Could you check a few things on this model? Use its own coordinates, in mm. Face numbers are marked on the shaded views. A direction names the side the tool comes from. Give positions to 0.01 mm unless a question says otherwise; leave off trailing zeros. Write each loop counter-clockwise with the first axis right and the second up, starting at its lowest first coordinate (ties: lowest second). Pieces come first, ordered by that corner, then holes. Notation, with made-up numbers: M 11.5,62.25 L 42.5,62.25 A24 ccw 42.5,86.25 Z; hole C 26.25,28 d2. An arc over 180 degrees is marked long. Answer as a JSON object with one key per item and string values. Group by question number.
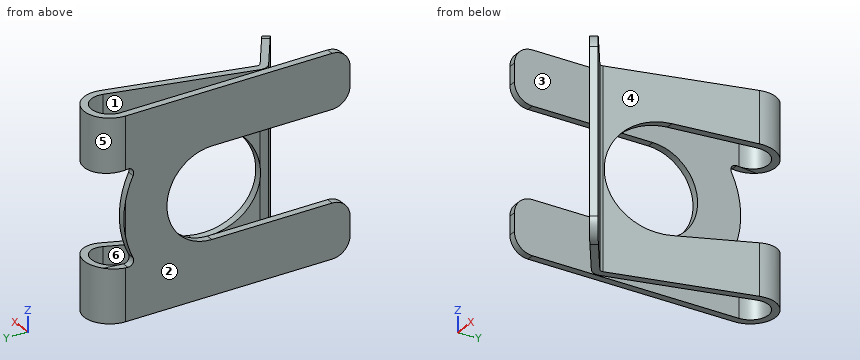
```python
from build123d import *

# Parameters (mm, degrees)
BOSS_EXTRUDE1_DEPTH      = 5.5
BOSS_EXTRUDE1_DEPTH_BACK = 5.5
CUT_EXTRUDE1_DEPTH       = 0.4
CUT_EXTRUDE2_DEPTH       = 3.8
CUT_EXTRUDE3_DEPTH       = 3.8
CUT_EXTRUDE4_DEPTH       = 0.4
CUT_EXTRUDE5_DEPTH       = 0.4
CUT_EXTRUDE6_DEPTH       = 0.4
CUT_EXTRUDE7_DEPTH       = 0.4
CUT_EXTRUDE8_DEPTH       = 0.8
CUT_EXTRUDE8_DEPTH_BACK  = 0.8


with BuildPart() as part:
    # Sketch1 → Boss-Extrude1 (new body, two sides)
    with BuildSketch(Plane.XY) as boss_extrude1_sk:
        with BuildLine():
            Line((0, 4.8), (0, -7.7))
            Line((0, -7.7), (0.4, -7.7))
            Line((0.4, -7.7), (0.4, 4.8))
            ThreePointArc((0.4, 4.8), (1.523848484, 5.79230114), (2.369323106, 4.554210017))
            Line((2.369323106, 4.554210017), (0.462124676, -2.967217351))
            ThreePointArc((0.462124676, -2.967217351), (0.483070792, -3.328406344), (0.707868785, -3.611888427))
            Line((0.707868785, -3.611888427), (3.611166589, -5.573025933))
            Line((3.611166589, -5.573025933), (3.835066425, -5.241561209))
            Line((3.835066425, -5.241561209), (0.931768621, -3.280423703))
            ThreePointArc((0.931768621, -3.280423703), (0.856835957, -3.185929675), (0.849853918, -3.065533344))
            Line((0.849853918, -3.065533344), (2.757052349, 4.455894023))
            ThreePointArc((2.757052349, 4.455894023), (1.573387877, 6.189221596), (0, 4.8))
        make_face()
    extrude(amount=BOSS_EXTRUDE1_DEPTH)
    extrude(boss_extrude1_sk.sketch, amount=-BOSS_EXTRUDE1_DEPTH_BACK)

    # Sketch2 → Cut-Extrude1 (cut)
    with BuildSketch(Plane(origin=(0, 0, 0), x_dir=(0, 0, -1), z_dir=(1, 0, 0))):
        with BuildLine():
            Line((-2.5, 0), (-2.5, -7.7))
            Line((-2.5, -7.7), (2.5, -7.7))
            Line((2.5, -7.7), (2.5, 0))
            ThreePointArc((2.5, 0), (0, 2.5), (-2.5, 0))
        make_face()
    extrude(amount=CUT_EXTRUDE1_DEPTH, mode=Mode.SUBTRACT)

    # Sketch3 → Cut-Extrude2 (cut)
    with BuildSketch(Plane(origin=(0.4, 0, 0), x_dir=(0, 0, -1), z_dir=(1, 0, 0))):
        with BuildLine():
            Line((2.989896199, 0.246009597), (2.5, 6.2))
            Line((2.5, 6.2), (-2.5, 6.2))
            Line((-2.5, 6.2), (-2.989896199, 0.246009597))
            ThreePointArc((-2.989896199, 0.246009597), (0, -3), (2.989896199, 0.246009597))
        make_face()
    extrude(amount=CUT_EXTRUDE2_DEPTH, mode=Mode.SUBTRACT)

    # Sketch4 → Cut-Extrude3 (cut)
    with BuildSketch(Plane(origin=(0.4, 0, 0), x_dir=(0, 0, -1), z_dir=(1, 0, 0))):
        with BuildLine():
            Line((2.62546601, 4.675139381), (2.5, 6.2))
            Line((2.5, 6.2), (-2.5, 6.2))
            Line((-2.5, 6.2), (-2.62546601, 4.675139381))
            ThreePointArc((-2.62546601, 4.675139381), (-2.494509309, 4.402012893), (-2.192256609, 4.382238122))
            ThreePointArc((-2.192256609, 4.382238122), (-6e-09, 4.9), (2.192256599, 4.382238127))
            ThreePointArc((2.192256599, 4.382238127), (2.494509304, 4.402012889), (2.62546601, 4.675139381))
        make_face()
    extrude(amount=-CUT_EXTRUDE3_DEPTH, mode=Mode.SUBTRACT)

    # Sketch5 → Cut-Extrude4 (cut)
    with BuildSketch(Plane(origin=(0, 0, 0), x_dir=(0, 0, -1), z_dir=(1, 0, 0))):
        with BuildLine():
            Line((-5.5, -7.7), (-4.5, -7.7))
            ThreePointArc((-4.5, -7.7), (-5.207106781, -7.407106781), (-5.5, -6.7))
            Line((-5.5, -6.7), (-5.5, -7.7))
        make_face()
    extrude(amount=CUT_EXTRUDE4_DEPTH, mode=Mode.SUBTRACT)

    # Sketch6 → Cut-Extrude5 (cut)
    with BuildSketch(Plane(origin=(0, 0, 0), x_dir=(0, 0, -1), z_dir=(1, 0, 0))):
        with BuildLine():
            Line((4.5, -7.7), (5.5, -7.7))
            Line((5.5, -7.7), (5.5, -6.7))
            ThreePointArc((5.5, -6.7), (5.207106781, -7.407106781), (4.5, -7.7))
        make_face()
    extrude(amount=CUT_EXTRUDE5_DEPTH, mode=Mode.SUBTRACT)

    # Sketch7 → Cut-Extrude6 (cut)
    with BuildSketch(Plane(origin=(0, 0, 0), x_dir=(0, 0, -1), z_dir=(1, 0, 0))):
        with BuildLine():
            Line((2.5, -7.7), (3.5, -7.7))
            ThreePointArc((3.5, -7.7), (2.792893219, -7.407106781), (2.5, -6.7))
            Line((2.5, -6.7), (2.5, -7.7))
        make_face()
    extrude(amount=CUT_EXTRUDE6_DEPTH, mode=Mode.SUBTRACT)

    # Sketch8 → Cut-Extrude7 (cut)
    with BuildSketch(Plane(origin=(0, 0, 0), x_dir=(0, 0, -1), z_dir=(1, 0, 0))):
        with BuildLine():
            Line((-3.5, -7.7), (-2.5, -7.7))
            Line((-2.5, -7.7), (-2.5, -6.7))
            ThreePointArc((-2.5, -6.7), (-2.792893219, -7.407106781), (-3.5, -7.7))
        make_face()
    extrude(amount=CUT_EXTRUDE7_DEPTH, mode=Mode.SUBTRACT)

    # Sketch9 → Cut-Extrude8 (cut, two sides)
    with BuildSketch(Plane(origin=(-1.229660553, -1.820408193, 0), x_dir=(0.82866181, -0.55974959, 0), z_dir=(0.55974959, 0.82866181, 0))) as cut_extrude8_sk:
        with BuildLine():
            Line((6.112336896, 4.5), (6.112336896, -4.5))
            ThreePointArc((6.112336896, -4.5), (5.819443678, -5.207106781), (5.112336896, -5.5))
            Line((5.112336896, -5.5), (5.112336896, -6.5))
            Line((5.112336896, -6.5), (7.112336896, -6.5))
            Line((7.112336896, -6.5), (7.112336896, 6.5))
            Line((7.112336896, 6.5), (5.112336896, 6.5))
            Line((5.112336896, 6.5), (5.112336896, 5.5))
            ThreePointArc((5.112336896, 5.5), (5.819443678, 5.207106781), (6.112336896, 4.5))
        make_face()
    extrude(amount=CUT_EXTRUDE8_DEPTH, mode=Mode.SUBTRACT)
    extrude(cut_extrude8_sk.sketch, amount=-CUT_EXTRUDE8_DEPTH_BACK, mode=Mode.SUBTRACT)


solid = part.part
```
1) Please list where these lines run through material, in increasing order: line 1 along X through (y, z) = (4.8, 4.3); line 2 along Z through (x, y) = (1.4, 0); line 3 along Z through (x, y) = (0.35, -2). Write a range as from..to.
2) For the marked faces 1, 2 and 3, which set-ups out of +Z, -Z, +X, -X, +Y, -Y let a thin tool reach every point of the face, with its end or its side?
3) If we section it at B-B, the plane z = 0: List the corners of the cut face in (x, y) for me.
4) I'm going to push a flat-ended pin straight in: pin 1 (5.5 mm diameter, centred on y = 0, z = -2.5, fed in from +X). Where does the tip first touch, or does it pass through?
5) If we section it at A-A, the plane y = -6: List the corners of the cut face in (x, z) for me, plus the area to 3 significant figures.
6) We'd pull the mould along X, two halves only. Please class the marked faces 4, 5 and 6: released by +X, released by -X, zero draft, split by the parting line, or undercut.
7) If we section it at D-D, the plane y = 4: List the corners of the cut face in (x, z) for me.
8) If we section it at C-C, the plane y = -0.25: List the corners of the cut face in (x, z) for me.
Taken from the geometry:
{
 "1": {"line 1": "0..0.4, 2.4..2.8", "line 2": "-5.5..-3, 3..5.5", "line 3": "-5.5..-2.5, 2.5..5.5"},
 "2": {"face 1": "+Z, -Z", "face 2": "+Z, -Z, -X, +Y, -Y", "face 3": "+Z, -Z, -Y"},
 "3": {"outline": "M 0,2.5 L 0.4,2.5 L 0.4,4.9 L 0,4.9 A1.4 ccw 0,4.8 Z; M 0.45,-3 A0.6 ccw 0.71,-3.61 L 3.61,-5.57 L 3.84,-5.24 L 0.93,-3.28 A0.2 cw 0.85,-3.07 L 0.87,-3 Z"},
 "4": {"pin 1": "x = 2.32"},
 "5": {"outline": "M 0,-5.5 L 0.4,-5.5 L 0.4,-2.5 L 0,-2.5 Z; M 0,2.5 L 0.4,2.5 L 0.4,5.5 L 0,5.5 Z", "area": "2.40 mm²"},
 "6": {"face 4": "released by +X", "face 5": "split by the parting line", "face 6": "undercut"},
 "7": {"outline": "M 0,-5.5 L 0.4,-5.5 L 0.4,5.5 L 0,5.5 Z; M 2.23,-5.5 L 2.64,-5.5 L 2.64,-2.68 L 2.23,-2.68 Z; M 2.23,2.68 L 2.64,2.68 L 2.64,5.5 L 2.23,5.5 Z"},
 "8": {"outline": "M 0,-5.5 L 0.4,-5.5 L 0.4,-2.5 L 0,-2.5 Z; M 0,2.5 L 0.4,2.5 L 0.4,5.5 L 0,5.5 Z; M 1.15,-5.5 L 1.56,-5.5 L 1.56,-2.99 L 1.15,-2.99 Z; M 1.15,2.99 L 1.56,2.99 L 1.56,5.5 L 1.15,5.5 Z"}
}
